Autodesk Inventor part; units mm, degrees
ref_plane "Work Plane2" through (0, -32.5, -80) normal (0, 0, -1) x (0, 1, 0)
ref_plane "Work Plane1" through (0, 0, 27.5) normal (0, 0, 1) x (1, 0, 0)
ref_plane "Work Plane3" through (0, 0, -200) normal (0, 0, -1) x (-1, 0, 0)
sketch "Sketch11" plane through (0, 0, 0) normal (1, 0, 0) x (0, 1, 0)
  line L0 (-309.4604, 0) -> (1517.2621, 0) construction
  line L1 (0, -249.7) -> (0, 98.2)
  circle A0 centre (0, 0) radius 32.5
  circle A1 centre (0, 0) radius 48.5
  line L2 (-30, -38.1084) -> (-30, -151.9615)
  line L3 (-30, -151.9615) -> (30, -151.9615)
  line L4 (30, -151.9615) -> (30, -38.1084)
  arc A2 (-30, -151.9615) -> (30, -151.9615) centre (0, -100) ccw
  arc A3 (30, -151.9615) -> (50, -133.1662) centre (0, -100) ccw
  line L5 (0, -180) -> (50, -180)
  line L6 (50, -180) -> (50, -133.1662)
  arc A4 (30, -38.1084) -> (35, -148.734) centre (1256.3018, -38.1084) ccw
  point P0 (-30, -151.9615)
  point P1 (0, -160)
  point P2 (0, -151.9615)
  point P3 (0, -185.7103)
  point P4 (0, -160)
  point P5 (0, -48.5)
  dimension "d77" = 65
  dimension "d78" = 97
  dimension "d79" = 60
  dimension "d85" = 20
  dimension "d86" = 20
  dimension "d87" = 60
  dimension "d89" = 35
  dimension "d90" = 160
extrude "Extrusion11" add sketch "Sketch11" along normal mid plane 60 contours L1 A1 L4 L3 | L4 A4 A3
revolve "Revolution1" add sketch "Sketch11" angle 180 mid plane about axis through (0, 0, -10) along (0, 0, 1) picked at (16.8404, -153.4348) contours L1 L3 A2
revolve "Revolution2" cut sketch "Sketch11" angle 360 about axis through (0, 0, -10) along (0, 0, 1) contours L1 A2 A3 L6 L5
mirror "Mirror1" about plane through (0, 0, 0) normal (0, 1, 0)
sketch "Sketch6" plane through (0, 0, 0) normal (1, 0, 0) x (0, 1, 0)
  circle A0 centre (0, 0) radius 32.5
  line L0 (-32.5, 0) -> (-32.5, -80)
  line L1 (-32.5, -80) -> (32.5, -80)
  line L2 (32.5, -80) -> (32.5, 0)
  line L3 (0, 0) -> (0, -80) construction
  line L4 (-32.5, -60) -> (32.5, -60)
  circle A1 centre (0, 0) radius 48.5
  point P0 (32.5, -36)
  point P1 (23.3184, -32.5)
  point P2 (0, -40)
  point P3 (-32.5, -36)
  dimension "d38" = 65
  dimension "d39" = 80
  dimension "d74" = 97
  dimension "d75" = 20
  dimension "d48" = 10
  dimension "d73" = 55
  dimension "d52" = 120
sketch "Sketch5" plane through (0, 0, -171) normal (0, 0, -1) x (-1, 0, 0)
  circle A0 centre (0, 0) radius 10
  point P0 (0, 0)
  dimension "d35" = 20
properties part number "shank_2"
Build history of the part. All positions in model axes, mm. Coordinates: 2 decimals unless noted, no trailing zeros. Order: outer loops, then holes, each group sorted by start corner. A loop starts at its lowest first (then second) coordinate and runs counter-clockwise, first axis right, second up. Notation, with made-up numbers: (-26, 23.5) -> (27, 23.5) arc R7 cw to (27, 30.5) -> close; hole circle Ø8 at (35.5, 57). An arc over 180 degrees is marked (long way). Answer in a Markdown table with one row per item. Add a question column.
Q1. Wall check: line 1 along Y through (x, z) = (-26, -45); line 2 along Y through (x, z) = (-16, -44); line 3 along Y through (x, z) = (22, -54.5). Give the ranges that are in metal, low to high. Write a range as [from, to].
Q2. Band-saw the part on A-A, the plane z = -46. List the corners of the cut face in (x, y), then the cut area to 3 significant figures.
Q3. Drop flat-ended pins along their axis: pin 1 (5 mm diameter, centred on x = 0, y = -7.5, fed in from +Z); pin 2 (1.5 mm diameter, centred on x = 12, z = -59, fed in from -Y); pin 3 (1 mm diameter, centred on x = -9.5, y = -13, fed in from -Z). Give the stop position or say it passes through.
Q4. Band-saw the part on C-C, the plane z = -110. List the corners of the cut face in (x, y), then the cut area to 3 significant figures.
Q5. Mould opens along Y. For faces 1 (the face through (-0.42, 0.453, -48.498)), 2 (the face through (-0.42, -31.216, -92.703)), 3 (the face through (-0.42, 31.286, -94.252)), 4 (the face through (-30, 0, -94)) say: +Y half, -Y half, draft (parallel to the pull), parting line (faces both ways), or undercut.
Q6. Band-saw the part on B-B, the plane z = -62. List the corners of the cut face in (x, y).
Answers follow:
| question | item | result |
|---|---|---|
| 1 | line 1 | [-30.02, -18.09], [18.09, 30.02] |
| 1 | line 2 | [-30.01, -20.4], [20.4, 30.01] |
| 1 | line 3 | [-30.11, 30.11] |
| 2 | outline | (-30, -30.03) -> (30, -30.03) -> (30, -15.37) -> (-30, -15.37) -> close; (-30, 15.37) -> (30, 15.37) -> (30, 30.03) -> (-30, 30.03) -> close |
| 2 | area | 1,760 mm^2 |
| 3 | pin 1 | z = -47.46 |
| 3 | pin 2 | y = -30.19 |
| 3 | pin 3 | z = -157.94 |
| 4 | outline | (-30, -32.11) -> (30, -32.11) -> (30, 32.11) -> (-30, 32.11) -> close |
| 4 | area | 3,850 mm^2 |
| 5 | face 1 | undercut |
| 5 | face 2 | -Y half |
| 5 | face 3 | +Y half |
| 5 | face 4 | draft |
| 6 | outline | (-30, -30.23) -> (30, -30.23) -> (30, 30.23) -> (-30, 30.23) -> close |
